```python
from build123d import *

# Parameters (mm, degrees)
BOSS_EXTRUDE1_DEPTH        = 10
CUT_EXTRUDE1_DEPTH         = 5
F_3_2_3_2_DIAMETER_HOLE1_D = 3.2
BOSS_EXTRUDE2_DEPTH        = 10
FILLET1_R                  = 3
FILLET2_R                  = 2
SKETCH21_R                 = 2.1
CUT_EXTRUDE2_DEPTH         = 36.522103107
SKETCH22_R                 = 3.5
CUT_EXTRUDE3_DEPTH         = 2.6
CUT_EXTRUDE6_DEPTH         = 2.5
SKETCH27_W                 = 2.6
SKETCH27_H                 = 3.5


with BuildPart() as part:
    # Sketch1 → Boss-Extrude1 (new body)
    with BuildSketch(Plane(origin=(0, 0, 0), x_dir=(1, 0, 0), z_dir=(0, 1, 0))):
        with BuildLine():
            ThreePointArc((-187.660784713, 29.722548358), (-190, 0), (-187.660784713, -29.722548358))
            Line((-187.660784713, -29.722548358), (-197.537668119, -31.286893008))
            ThreePointArc((-197.537668119, -31.286893008), (-200, 0), (-197.537668119, 31.286893008))
            Line((-197.537668119, 31.286893008), (-187.660784713, 29.722548358))
        make_face()
        with BuildLine():
            ThreePointArc((-197.537668119, -31.286893008), (-200, 0), (-197.537668119, 31.286893008))
            Line((-197.537668119, 31.286893008), (-201.982265652, 31.990848101))
            ThreePointArc((-201.982265652, 31.990848101), (-204.5, 0), (-201.982265652, -31.990848101))
            Line((-201.982265652, -31.990848101), (-197.537668119, -31.286893008))
        make_face()
        with BuildLine():
            Line((-184.697719691, 29.253244963), (-187.660784713, 29.722548358))
            ThreePointArc((-187.660784713, 29.722548358), (-190, 0), (-187.660784713, -29.722548358))
            Line((-187.660784713, -29.722548358), (-184.697719691, -29.253244963))
            ThreePointArc((-184.697719691, -29.253244963), (-187, 0), (-184.697719691, 29.253244963))
        make_face()
    extrude(amount=BOSS_EXTRUDE1_DEPTH)

    # Sketch15 → Cut-Extrude1 (cut)
    with BuildSketch(Plane(origin=(0, 10, 0), x_dir=(1, 0, 0), z_dir=(0, 1, 0))):
        with BuildLine():
            Line((-199.749843554, 10), (-189.73665961, 10))
            ThreePointArc((-189.73665961, 10), (-188.956218405, 19.88837666), (-187.660784713, 29.722548358))
            Line((-187.660784713, 29.722548358), (-197.537668119, 31.286893008))
            ThreePointArc((-197.537668119, 31.286893008), (-198.928692466, 20.673057674), (-199.749843554, 10))
        make_face()
        with BuildLine():
            ThreePointArc((-187.660784713, -29.722548358), (-188.956218405, -19.88837666), (-189.73665961, -10))
            Line((-189.73665961, -10), (-199.749843554, -10))
            ThreePointArc((-199.749843554, -10), (-198.928692466, -20.673057674), (-197.537668119, -31.286893008))
            Line((-197.537668119, -31.286893008), (-187.660784713, -29.722548358))
        make_face()
    extrude(amount=-CUT_EXTRUDE1_DEPTH, mode=Mode.SUBTRACT)

    # Ø3.2 (3.2) Diameter Hole1 (through all)
    with Locations(Plane(origin=(0, 0, 0), x_dir=(-1, 0, 0), z_dir=(0, -1, 0))):
        with Locations((194.257966128, -16.995369836), (194.257966128, 16.995369836)):
            Hole(F_3_2_3_2_DIAMETER_HOLE1_D / 2)

    # Sketch19 → Boss-Extrude2 (add)
    with BuildSketch(Plane(origin=(0, 0, 0), x_dir=(1, 0, 0), z_dir=(0, 1, 0))):
        with BuildLine():
            Line((-185.102830261, -12.132280472), (-186.599618646, -12.230385166))
            ThreePointArc((-186.599618646, -12.230385166), (-187, 0), (-186.599618646, 12.230385166))
            Line((-186.599618646, 12.230385166), (-185.102830261, 12.132280472))
            ThreePointArc((-185.102830261, 12.132280472), (-185.5, 0), (-185.102830261, -12.132280472))
        make_face()
    extrude(amount=BOSS_EXTRUDE2_DEPTH)

    # Fillet1
    # the kernel refuses this fillet: 3 mm, written as the material it adds along each edge
    with BuildSketch(Plane(origin=(-186.599618646, 0, -12.230385166), x_dir=(0.07241784502459461, 0, -0.9973743809232287), z_dir=(0, 1, 0))) as fillet1_piece_1:
        with BuildLine():
            CenterArc((2.608644701, -2.999925838), FILLET1_R, 89.597127862, 60.403689883)
            Line((0.010547081, -1.499962919), (-0.041414871, -1.469963661))
            ThreePointArc((-0.041414871, -1.469963661), (-0.054724976, -0.750403343), (-0.059998517, -0.000421883))
            Line((-0.059998517, -0.000421883), (-0.000421883, 0.059998517))
            ThreePointArc((-0.000421883, 0.059998517), (1.314869431, 0.064622735), (2.630160746, 0.059998517))
            Line((2.630160746, 0.059998517), (2.629738863, 0))
        make_face()
    extrude(amount=10)
    with BuildSketch(Plane(origin=(-186.599618646, 0, 12.230385166), x_dir=(0.0724178450245846, 0, 0.9973743809232295), z_dir=(0, 1, 0))) as fillet1_piece_2:
        with BuildLine():
            CenterArc((2.608644701, 2.999925838), FILLET1_R, 209.999182255, 60.403689883)
            Line((0.010547081, 1.499962919), (-0.041414871, 1.469963661))
            ThreePointArc((-0.041414871, 1.469963661), (-0.054724976, 0.750403343), (-0.059998517, 0.000421883))
            Line((-0.059998517, 0.000421883), (-0.000421883, -0.059998517))
            ThreePointArc((-0.000421883, -0.059998517), (1.314869431, -0.064622735), (2.630160746, -0.059998517))
            Line((2.630160746, -0.059998517), (2.629738863, 0))
        make_face()
    extrude(amount=10)

    # Fillet2
    fillet2_edges = [part.edges().sort_by_distance(p)[0] for p in [
        (-201.982265652, 5, 31.990848101),
        (-201.982265652, 5, -31.990848101),
        (-184.697719691, 5, -29.253244963),
        (-184.697719691, 5, 29.253244963),
    ]]
    fillet(fillet2_edges, radius=FILLET2_R)

    # Sketch21 → Cut-Extrude2 (cut, through all)
    with BuildSketch(Plane(origin=(-197.5, 0, 0), x_dir=(0, 0, -1), z_dir=(1, 0, 0))):
        with Locations((0, 10)):
            Circle(SKETCH21_R)
    extrude(amount=CUT_EXTRUDE2_DEPTH, mode=Mode.SUBTRACT)

    # Sketch22 → Cut-Extrude3 (cut)
    with BuildSketch(Plane(origin=(-197.5, 0, 0), x_dir=(0, 0, -1), z_dir=(1, 0, 0))):
        with Locations((0, 10)):
            Circle(SKETCH22_R)
    extrude(amount=CUT_EXTRUDE3_DEPTH, mode=Mode.SUBTRACT)

    # Sketch26 → Cut-Extrude6 (cut)
    with BuildSketch(Plane.XZ):
        with BuildLine():
            Line((-199.997133786, -31.676434101), (-186.662644351, -29.564458455))
            ThreePointArc((-186.662644351, -29.564458455), (-185.363721979, -28.773196969), (-184.996936421, -27.297133819))
            ThreePointArc((-184.996936421, -27.297133819), (-185.807261228, -21.087002508), (-186.409178624, -14.853219336))
            ThreePointArc((-186.409178624, -14.853219336), (-186.123110766, -13.316498702), (-185.102830261, -12.132280472))
            ThreePointArc((-185.102830261, -12.132280472), (-185.5, 0), (-185.102830261, 12.132280472))
            ThreePointArc((-185.102830261, 12.132280472), (-186.123110766, 13.316498702), (-186.409178624, 14.853219336))
            ThreePointArc((-186.409178624, 14.853219336), (-185.807261228, 21.087002508), (-184.996936421, 27.297133819))
            ThreePointArc((-184.996936421, 27.297133819), (-185.363721979, 28.773196969), (-186.662644351, 29.564458455))
            Line((-186.662644351, 29.564458455), (-199.997133786, 31.676434101))
            ThreePointArc((-199.997133786, 31.676434101), (-201.493549275, 31.313266322), (-202.288373113, 29.994401197))
            ThreePointArc((-202.288373113, 29.994401197), (-204.5, 0), (-202.288373113, -29.994401197))
            ThreePointArc((-202.288373113, -29.994401197), (-201.493549275, -31.313266322), (-199.997133786, -31.676434101))
        make_face()
    extrude(amount=-CUT_EXTRUDE6_DEPTH, mode=Mode.SUBTRACT)

    # Sketch27 → Cut-Revolve3 (revolve, cut)
    with BuildSketch(Plane(origin=(0, 10, 0), x_dir=(1, 0, 0), z_dir=(0, 1, 0))):
        with Locations((-186.766978193, 1.75)):
            Rectangle(SKETCH27_W, SKETCH27_H)
    revolve(axis=Axis((-197.5, 10, 0), (1, 0, 0)), mode=Mode.SUBTRACT)


solid = part.part
```
Part model, mm, in its own coordinate system. A direction names the side the tool comes from. Round coordinates to 2 decimals unless told otherwise and drop trailing zeros. Write each loop counter-clockwise with the first axis right and the second up, starting at its lowest first coordinate (ties: lowest second). Pieces come first, ordered by that corner, then holes.
Item 1: Which spindle directions (+Z, -Z, +X, -X, +Y, -Y) get a long thin tool onto all of the face, cutting with end or side? Do faces 4 (the cylindrical face through (-188.94, 7.54, 20.03)), 5 (the flat face through (-188.067, 7, 0)), 6 (the flat face through (-194, 5, 20)), 7 (the cylindrical face through (-185.817, 6.198, -21)). Say none if no direction does.
Results:
face 4: +Z, +Y
face 5: +X, +Y
face 6: +Y
face 7: +X, +Y, -Y
Item 2: Drop flat-ended pins along their axis: pin 1 Ø3.5 at (x, z) = (-194.26, 17) entering from -Y; pin 2 Ø1.8 at (y, z) = (7.5, 1.5) entering from +X; pin 3 Ø2.5 at (x, y) = (-192.5, 7.5) entering from +Z; pin 4 Ø2 at (x, y) = (-188, 5) entering from -Z. Give the stop position or say it passes through.
Results:
pin 1: stops at y = 2.5
pin 2: stops at x = -185.48
pin 3: stops at z = 10
pin 4: stops at z = -29.93
Item 3: Probe L1, parallel to Z at x = -196.25, y = 9.75; L2, parallel to Z at x = -193.5, y = 4; L3, parallel to X at y = 8, z = -1. List the from-to ranges inside material, lowest first.
Results:
L1: z = -10 to -3.49, 3.49 to 10
L2: z = -30.65 to -18.4, -15.59 to 15.59, 18.4 to 30.65
L3: x = -204.5 to -197.5, -194.9 to -188.07
Item 4: Cut at B-B, the plane y = 4. Give the cut face in (x, z).
Results:
outline: (-202.29, -29.99) arc R2 ccw to (-200, -31.68) - (-186.66, -29.56) arc R2 ccw to (-185, -27.3) arc R187 cw to (-186.41, -14.85) arc R3 cw to (-185.1, -12.13) arc R185.5 cw to (-185.1, 12.13) arc R3 cw to (-186.41, 14.85) arc R187 cw to (-185, 27.3) arc R2 ccw to (-186.66, 29.56) - (-200, 31.68) arc R2 ccw to (-202.29, 29.99) arc R204.5 ccw to start; hole circle Ø3.2 at (-194.26, -17); hole circle Ø3.2 at (-194.26, 17)
Item 5: Cut at C-C, the plane z = 0. Give the cut face in (x, y), plus the area to 3 significant figures.
Results:
outline: (-204.5, 2.5) - (-185.5, 2.5) - (-185.5, 6.5) - (-188.07, 6.5) - (-188.07, 7.9) - (-194.9, 7.9) - (-194.9, 6.5) - (-197.5, 6.5) - (-197.5, 10) - (-204.5, 10) - close
area: 110 mm2
Item 6: Cut at A-A, the plane z = 16. Give the cut face in (x, y).
Results:
outline: (-203.87, 2.5) - (-195.51, 2.5) - (-195.51, 5) - (-199.36, 5) - (-199.36, 10) - (-203.87, 10) - close; (-193.01, 2.5) - (-186.31, 2.5) - (-186.31, 10) - (-189.33, 10) - (-189.33, 5) - (-193.01, 5) - close
Item 7: Two-plate mould, pull along X, no slides. Class faces 1 (the cylindrical face through (-185.797, 6.198, 21.174)), 2 (the cylindrical face through (-188.97, 7.54, -19.75)), 3 (the flat face through (-199, 10, 0)): +X half, -X half, draft (parallel to the pull), parting line (faces both ways), or undercut.
Results:
face 1: +X half
face 2: undercut
face 3: draft
